Work out the finished part from the listing and answer in its coordinate system (mm). Face numbers are marked on the shaded views. Coordinates: 2 decimals unless noted, no trailing zeros. Order: outer loops, then holes, each group sorted by start corner. A loop starts at its lowest first (then second) coordinate and runs counter-clockwise, first axis right, second up.
```python
from build123d import *

# Parameters (mm, degrees)
BOSS_EXTRUDE1_DEPTH = 20
SKETCH2_R           = 10
BOSS_EXTRUDE2_DEPTH = 5
BOSS_EXTRUDE3_START = 5
SKETCH3_R           = 10
BOSS_EXTRUDE3_DEPTH = 5
SKETCH4_R           = 10
BOSS_EXTRUDE4_DEPTH = 5


with BuildPart() as part:
    # Sketch1 → Boss-Extrude1 (new body)
    with BuildSketch(Plane.XY):
        with BuildLine():
            Line((-46.135379716, 14.647544511), (153.864620284, 14.647544511))
            ThreePointArc((153.864620284, 14.647544511), (160.935688096, 11.718612322), (163.864620284, 4.647544511))
            ThreePointArc((163.864620284, 4.647544511), (160.935688096, -2.423523301), (153.864620284, -5.352455489))
            Line((153.864620284, -5.352455489), (-46.135379716, -5.352455489))
            ThreePointArc((-46.135379716, -5.352455489), (-53.206447528, -2.423523301), (-56.135379716, 4.647544511))
            ThreePointArc((-56.135379716, 4.647544511), (-53.206447528, 11.718612322), (-46.135379716, 14.647544511))
        make_face()
    extrude(amount=BOSS_EXTRUDE1_DEPTH)

    # Sketch2 → Boss-Extrude2 (add)
    with BuildSketch(Plane.XY.offset(20)):
        with Locations(Location((-46.135379716, 4.647544511, 0), (0, 0, 270))):
            Circle(SKETCH2_R)
    extrude(amount=BOSS_EXTRUDE2_DEPTH)

    # Sketch3 → Boss-Extrude3 (add)
    with BuildSketch(Plane(origin=(0, 0, 0), x_dir=(-1, 0, 0), z_dir=(0, 0, -1)).offset(BOSS_EXTRUDE3_START)):
        with Locations((46.135379716, 4.647544511)):
            Circle(SKETCH3_R)
    extrude(amount=-BOSS_EXTRUDE3_DEPTH)

    # Sketch4 → Boss-Extrude4 (add)
    with BuildSketch(Plane.XY.offset(20)):
        with Locations(Location((153.864620284, 4.647544511, 0), (0, 0, 90))):
            Circle(SKETCH4_R)
    extrude(amount=BOSS_EXTRUDE4_DEPTH)


solid = part.part
```
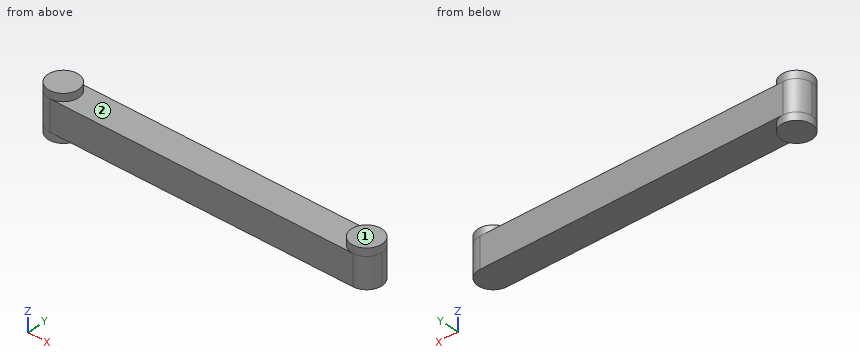
1. Flat-ended cylindrical pins translate along their axes: pin 1 (10 mm diameter, centred on x = 139.5, y = 12, fed in from -Z); pin 2 (8 mm diameter, centred on x = 40.5, z = -0.5, fed in from -Y); pin 3 (10 mm diameter, centred on x = 43.5, y = 1.5, fed in from +Z). Find the tip coordinate at first contact, or state that the pin passes through.
2. The part is cut by section C-C (x = -20.5). Determine the outline of the cut face in (y, z), plus the area to 3 significant figures.
3. The part is cut by section A-A (y = 11.75). Determine the outline of the cut face in (x, z), plus the area to 3 significant figures.
4. Consider probe 1 along Z at (x, y) = (75.5, 0.5); probe 2 along Y at (x, z) = (154.5, 20.25); probe 3 along X at (y, z) = (10, 23.5). Determine where each line is inside the solid, lowest interval first.
5. The part is cut by section D-D (y = 0). Determine the outline of the cut face in (x, z), plus the area to 3 significant figures.
6. The part is cut by section B-B (z = 15.75). Determine the outline of the cut face in (x, y).
7. The mould has two halves that part along X. Classify the marked faces 1 and 2: released by +X, released by -X, zero draft, split by the parting line, or undercut.
Worked out:
1. pin 1: stops at z = 0
1. pin 2: stops at y = -5.35
1. pin 3: stops at z = 20
2. outline: (-5.35, 0) - (14.65, 0) - (14.65, 20) - (-5.35, 20) - close
2. area: 400 mm2
3. outline: (-53.17, -5) - (-39.1, -5) - (-39.1, 0) - (160.9, 0) - (160.9, 25) - (146.83, 25) - (146.83, 20) - (-39.1, 20) - (-39.1, 25) - (-53.17, 25) - close
3. area: 4,490 mm2
4. probe 1: z = 0 to 20
4. probe 2: y = -5.33 to 14.63
4. probe 3: x = -54.58 to -37.69, 145.42 to 162.31
5. outline: (-54.99, -5) - (-37.28, -5) - (-37.28, 0) - (162.72, 0) - (162.72, 25) - (145.01, 25) - (145.01, 20) - (-37.28, 20) - (-37.28, 25) - (-54.99, 25) - close
5. area: 4,620 mm2
6. outline: (-46.14, -5.35) - (153.86, -5.35) arc R10 ccw to (153.86, 14.65) - (-46.14, 14.65) arc R10 ccw to start
7. face 1: zero draft
7. face 2: undercut
